Build history of the part. All positions in model axes, mm. Face numbers are marked on the shaded views. A direction names the side the tool comes from. Round coordinates to 2 decimals unless told otherwise and drop trailing zeros. Loops run counter-clockwise (first coordinate to the right, second up) from the corner with the lowest first, then second, coordinate; pieces in that order, holes last. Notation, with made-up numbers: (-1, -5.5) -> (47, -5.5) arc R16 cw to (47, 12.5) -> close; hole circle Ø4 at (28.25, 32.25). An arc over 180 degrees is marked (long way). Put each result on its own line as item: value. Start each with the question number.
Item 1: Cut at A-A, the plane y = 171.5. List the corners of the cut face in (x, z), plus the area to 3 significant figures.
Item 2: Pull direction Y, two halves, no side cores. Call the marked faces 1, 2 and 3: +Y half, -Y half, draft (parallel to the pull), parting line (faces both ways), or undercut.
Item 3: Flat gauge pin, fed straight in: pin 1 Ø1.5 at (x, z) = (0.5, 3) entering from -Y. Where does the tip first touch, or does it go through?
Item 4: Cut at B-B, the plane z = 4.5. List the corners of the cut face in (x, y).
Item 5: Tool access for the marked faces 4 and 5: list every direction of +Z, -Z, +X, -X, +Y, -Y with a clear straight run to the whole face (end or side of a thin tool).
Item 6: Drill centre lines: probe 1 along X at (y, z) = (109, 4.45); probe 2 along Y at (x, z) = (-7, 3); probe 3 along Y at (x, z) = (21.5, 3.05). Where is each one in solid material? Low to high. Write a range as [from, to].
Item 7: Cut at C-C, the plane y = 158.5. List the corners of the cut face in (x, z).
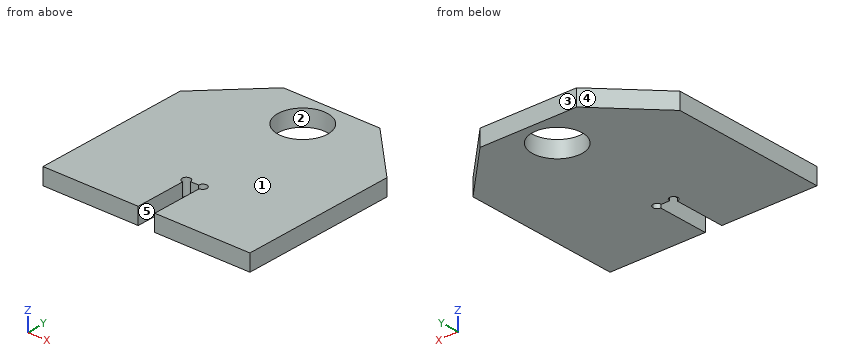
```python
from build123d import *

# Parameters (mm, degrees)
SKETCH1_R           = 9
BOSS_EXTRUDE1_DEPTH = 6


with BuildPart() as part:
    # Sketch1 → Boss-Extrude1 (new body)
    with BuildSketch(Plane.XY):
        with BuildLine():
            Line((3, 100), (37.5, 100))
            Line((37.5, 100), (37.5, 157))
            Line((37.5, 157), (17.5, 177))
            Line((17.5, 177), (-17.5, 177))
            Line((-17.5, 177), (-37.5, 157))
            Line((-37.5, 157), (-37.5, 100))
            Line((-37.5, 100), (-3, 100))
            Line((-3, 100), (-3, 118.5))
            ThreePointArc((-3, 118.5), (-4.060660172, 121.060660172), (-1.5, 120))
            Line((-1.5, 120), (1.5, 120))
            ThreePointArc((1.5, 120), (3, 121.5), (4.5, 120))
            ThreePointArc((4.5, 120), (4.060660172, 118.939339828), (3, 118.5))
            Line((3, 118.5), (3, 100))
        make_face()
        with Locations((8.6489e-05, 165)):
            Circle(SKETCH1_R, mode=Mode.SUBTRACT)
    extrude(amount=BOSS_EXTRUDE1_DEPTH)


solid = part.part
```
Reply:
1. outline: (-23, 0) -> (-6.22, 0) -> (-6.22, 6) -> (-23, 6) -> close; (6.23, 0) -> (23, 0) -> (23, 6) -> (6.23, 6) -> close
1. area: 201 mm^2
2. face 1: draft
2. face 2: undercut
2. face 3: +Y half
3. pin 1: stops at y = 120
4. outline: (-37.5, 100) -> (-3, 100) -> (-3, 118.5) arc R1.5 cw (long way) to (-1.5, 120) -> (1.5, 120) arc R1.5 cw (long way) to (3, 118.5) -> (3, 100) -> (37.5, 100) -> (37.5, 157) -> (17.5, 177) -> (-17.5, 177) -> (-37.5, 157) -> close; hole circle Ø18 at (0, 165)
5. face 4: +Z, -Z, -X, +Y
5. face 5: +Z, -Z, -Y
6. probe 1: x = [-37.5, -3], [3, 37.5]
6. probe 2: y = [100, 159.34], [170.66, 177]
6. probe 3: y = [100, 173]
7. outline: (-36, 0) -> (-6.22, 0) -> (-6.22, 6) -> (-36, 6) -> close; (6.23, 0) -> (36, 0) -> (36, 6) -> (6.23, 6) -> close
